Drawing for the job (mm, zero at the part's lowest x, y, z). A direction names the side the tool comes from. Round coordinates to 2 decimals unless told otherwise and drop trailing zeros. Order: outer loops, then holes, each group sorted by start corner. A loop starts at its lowest first (then second) coordinate and runs counter-clockwise, first axis right, second up. Notation, with made-up numbers: (-39, -30) - (-32, -30) arc R5 cw to (-32, -22) - close; hole circle Ø5 at (-4, 46.5). An arc over 180 degrees is marked (long way). Answer as a JSON object with one key per item and string values.
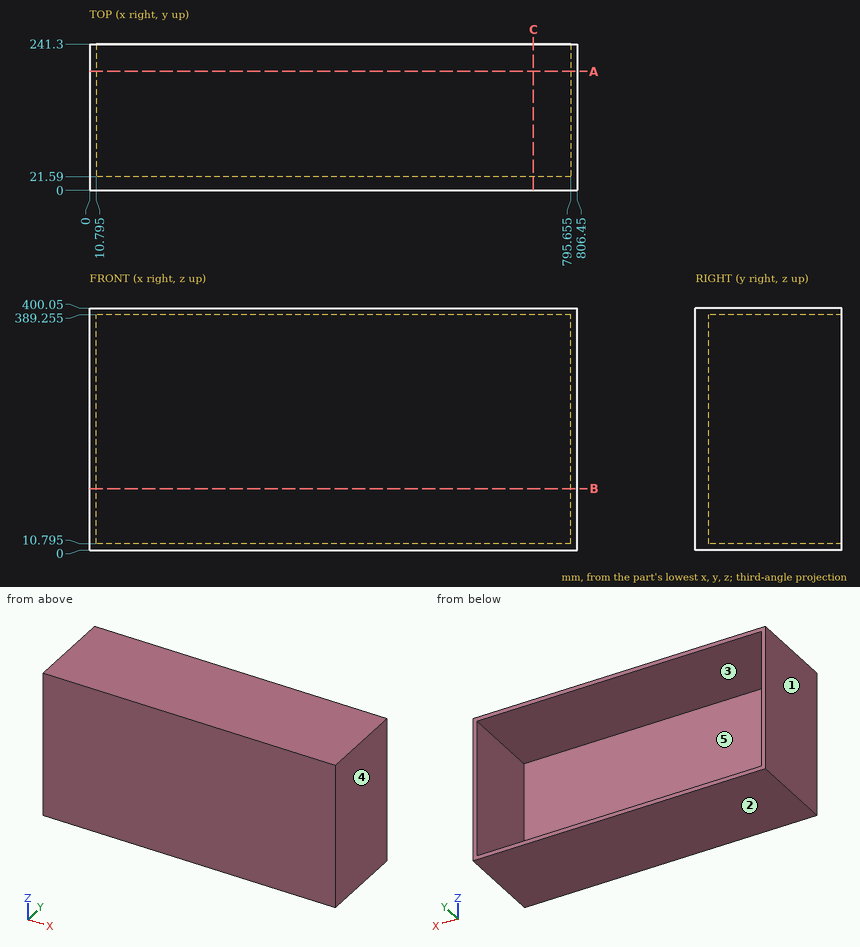
Item 1: Drop a flat-ended pin along its axis: P1, Ø12, axis at x = 418.5, z = 84.5, coming from the +Y side. Give the stop position or say it passes through.
Taken from the geometry:
{"P1": "y = 21.59"}
Item 2: Cut at A-A (y = 196). Write the cut outline in (x, z) (3 decimals).
Taken from the geometry:
{"outline": "(0, 0) - (806.45, 0) - (806.45, 400.05) - (0, 400.05) - close; hole (10.795, 10.795) - (795.655, 10.795) - (795.655, 389.255) - (10.795, 389.255) - close"}
Item 3: Cut at C-C (x = 733.5). Write the cut outline in (y, z) (3 decimals).
Taken from the geometry:
{"outline": "(0, 0) - (241.3, 0) - (241.3, 10.795) - (21.59, 10.795) - (21.59, 389.255) - (241.3, 389.255) - (241.3, 400.05) - (0, 400.05) - close"}
Item 4: Probe L1, parallel to X at y = 217.5, z = 225 (3 decimals); L2, parallel to Z at x = 649, y = 86.5 (3 decimals); L3, parallel to Y at x = 773.5, z = 211. List the from-to ranges inside material, lowest first. Write a range as from..to.
Taken from the geometry:
{"L1": "0..10.795, 795.655..806.45", "L2": "0..10.795, 389.255..400.05", "L3": "0..21.59"}
Item 5: Tool access for the marked faces 4 and 5: list every direction of +Z, -Z, +X, -X, +Y, -Y with a clear straight run to the whole face (end or side of a thin tool).
Taken from the geometry:
{"face 4": "+Z, -Z, +X, +Y, -Y", "face 5": "+Y"}
Item 6: Two-plate mould, pull along X, no slides. Class the marked faces 1, 2 and 3: pulls with the +X half, pulls with the -X half, needs draft (parallel to the pull), parting line crosses it, or undercut.
Taken from the geometry:
{"face 1": "pulls with the -X half", "face 2": "needs draft", "face 3": "undercut"}
Item 7: Cut at B-B (z = 101.5). Write the cut outline in (x, y) (3 decimals), plus the area to 3 significant figures.
Taken from the geometry:
{"outline": "(0, 0) - (806.45, 0) - (806.45, 241.3) - (795.655, 241.3) - (795.655, 21.59) - (10.795, 21.59) - (10.795, 241.3) - (0, 241.3) - close", "area": "22,200 mm2"}
